from build123d import *

# Parameters (mm, degrees)
F0_R     = 7.4
F0_R_2   = 2.5
F1_DEPTH = 4
F0_R_3   = 7.9
F2_DEPTH = 8.5
F3_DEPTH = 6.65


with BuildPart() as f1:
    # F0 (on Right) → F1 (new body)
    with BuildSketch(Plane.YZ):
        Circle(F0_R)
        Circle(F0_R_2, mode=Mode.SUBTRACT)
    extrude(amount=F1_DEPTH)

    # F0 (on Right) → F2 (join)
    with BuildSketch(Plane.YZ):
        Circle(F0_R_3)
        Circle(F0_R, mode=Mode.SUBTRACT)
    extrude(amount=F2_DEPTH)

    # F0 (on Right) → F3 (join)
    with BuildSketch(Plane.YZ):
        Circle(F0_R_2)
    extrude(amount=F3_DEPTH)


solid = f1.part
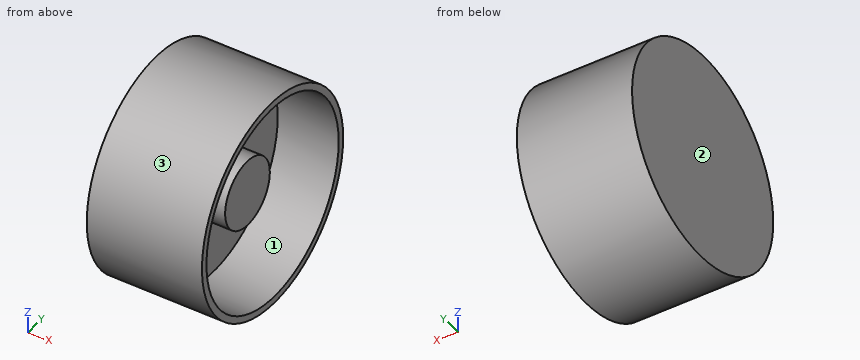
Verification items for the finished model (mm, model axes). Face numbers are marked on the shaded views. Give positions to 0.01 mm unless a question says otherwise; leave off trailing zeros. Loops run counter-clockwise (first coordinate to the right, second up) from the corner with the lowest first, then second, coordinate; pieces in that order, holes last.
1) Thickness scan on line 1 along X through (y, z) = (-7, -0.25); line 2 along Z through (x, y) = (7.25, 2.5); line 3 along Z through (x, y) = (5.5, -5). Record the ranges inside material, lowest first.
2) Sectioned sample at C-C, the plane x = 7. Enter the section's corners in (y, z), then the cut area to 3 significant figures.
3) Sectioned sample at B-B, the plane y = 1.25. Enter the section's corners in (x, z).
4) Draft check along Z on the marked faces 1, 2 and 3. Enter one of: pulls with the +Z half, pulls with the -Z half, needs draft (parallel to the pull), parting line crosses it, or undercut.
5) Sectioned sample at D-D, the plane x = 3.5. Enter the section's corners in (y, z).
6) Sectioned sample at A-A, the plane z = 0. Enter the section's corners in (x, y), then the cut area to 4 significant figures.
7) Depth check by flat-ended pin: pin 1 Ø5 at (y, z) = (-2, 0.5) entering from +X; pin 2 Ø1 at (x, z) = (1, -1.5) entering from +Y; pin 3 Ø1.5 at (x, z) = (5.5, 5.5) entering from +Y. Enter the tip coordinate at first touch or a pass-through.
Answers:
1. line 1: x = 0 to 4
1. line 2: z = -7.49 to -6.96, 6.96 to 7.49
1. line 3: z = -6.12 to -5.46, 5.46 to 6.12
2. outline: circle Ø15.8 at (0, 0); hole circle Ø14.8 at (0, 0)
2. area: 24.0 mm2
3. outline: (0, -7.8) - (8.5, -7.8) - (8.5, -7.29) - (4, -7.29) - (4, -2.17) - (6.65, -2.17) - (6.65, 2.17) - (4, 2.17) - (4, 7.29) - (8.5, 7.29) - (8.5, 7.8) - (0, 7.8) - close
4. face 1: undercut
4. face 2: needs draft
4. face 3: parting line crosses it
5. outline: circle Ø15.8 at (0, 0)
6. outline: (0, -7.9) - (8.5, -7.9) - (8.5, -7.4) - (4, -7.4) - (4, -2.5) - (6.65, -2.5) - (6.65, 2.5) - (4, 2.5) - (4, 7.4) - (8.5, 7.4) - (8.5, 7.9) - (0, 7.9) - close
6. area: 80.95 mm2
7. pin 1: stops at x = 6.65
7. pin 2: stops at y = 7.84
7. pin 3: stops at y = 6.31
